Geometry: final body of the model. Coordinates: model frame, mm. Face numbers are marked on the shaded views. A direction names the side the tool comes from. Round coordinates to 2 decimals unless told otherwise and drop trailing zeros. Loops run counter-clockwise (first coordinate to the right, second up) from the corner with the lowest first, then second, coordinate; pieces in that order, holes last. Notation, with made-up numbers: (59, 22.25) -> (106, 22.25) arc R22 cw to (106, 53.25) -> close; hole circle Ø5 at (9, 76.5). An arc over 180 degrees is marked (long way). Answer in a Markdown table with one row per item.
```python
from build123d import *

# Parameters (mm, degrees)
SKETCH2_R           = 1.625
BOSS_EXTRUDE1_DEPTH = 10
SKETCH3_R           = 2.875
CUT_EXTRUDE1_DEPTH  = 1.5
SKETCH4_W           = 42
SKETCH4_H           = 5
BOSS_EXTRUDE2_DEPTH = 30
SKETCH5_W           = 42
SKETCH5_H           = 5
BOSS_EXTRUDE3_DEPTH = 8
CUT_EXTRUDE2_REACH  = 44
SKETCH6_W           = 12.701613413
SKETCH6_H           = 5
CUT_EXTRUDE3_REACH  = 7
SKETCH8_R           = 1.625
SKETCH9_R           = 2.875
CUT_EXTRUDE4_DEPTH  = 1.5
CUT_EXTRUDE5_DEPTH  = 35


with BuildPart() as part:
    # Sketch2 → Boss-Extrude1 (new body)
    with BuildSketch(Plane(origin=(0, 0, 0), x_dir=(1, 0, 0), z_dir=(0, 1, 0))):
        Polygon((-21, 4.97717469), (-21, -4.97717469), (21, -4.97717469), (21, 4.97717469), (21, 12.724438723), (-21, 12.724438723), align=None)
        with Locations((-15.475, 0.182409544)):
            Circle(SKETCH2_R, mode=Mode.SUBTRACT)
        with Locations((15.475, 0.182409544)):
            Circle(SKETCH2_R, mode=Mode.SUBTRACT)
    extrude(amount=BOSS_EXTRUDE1_DEPTH)

    # Sketch3 → Cut-Extrude1 (cut)
    with BuildSketch(Plane(origin=(0, 10, 0), x_dir=(1, 0, 0), z_dir=(0, 1, 0))):
        with Locations((-15.475, 0.182409544)):
            Circle(SKETCH3_R)
        with Locations((15.475, 0.182409544)):
            Circle(SKETCH3_R)
    extrude(amount=-CUT_EXTRUDE1_DEPTH, mode=Mode.SUBTRACT)

    # Sketch4 → Boss-Extrude2 (add)
    with BuildSketch(Plane.XZ):
        with Locations((0, -10.224438723)):
            Rectangle(SKETCH4_W, SKETCH4_H)
    extrude(amount=BOSS_EXTRUDE2_DEPTH)

    # Sketch5 → Boss-Extrude3 (add)
    with BuildSketch(Plane(origin=(0, 0, -12.724438723), x_dir=(-1, 0, 0), z_dir=(0, 0, -1))):
        with Locations((0, -27.5)):
            Rectangle(SKETCH5_W, SKETCH5_H)
    extrude(amount=BOSS_EXTRUDE3_DEPTH)

    # Sketch6 → Cut-Extrude2 (cut, up to next)
    with BuildSketch(Plane.ZY.offset(21), mode=Mode.PRIVATE) as cut_extrude2_sk1:
        with Locations((-1.373632017, 2.5)):
            Rectangle(SKETCH6_W, SKETCH6_H)
    cut_extrude2_tool1 = extrude(cut_extrude2_sk1.sketch, amount=-CUT_EXTRUDE2_REACH, mode=Mode.PRIVATE) & part.part
    add(cut_extrude2_tool1.solids().sort_by_distance((-21, 2.5, -1.373632))[0], mode=Mode.SUBTRACT)

    # Sketch8 → Cut-Extrude3 (cut, up to next)
    with BuildSketch(Plane(origin=(0, -25, 0), x_dir=(1, 0, 0), z_dir=(0, 1, 0)), mode=Mode.PRIVATE) as cut_extrude3_sk1:
        with Locations((-15.475, 16.884966607)):
            Circle(SKETCH8_R)
    cut_extrude3_tool1 = extrude(cut_extrude3_sk1.sketch, amount=-CUT_EXTRUDE3_REACH, mode=Mode.PRIVATE) & part.part
    add(cut_extrude3_tool1.solids().sort_by_distance((-15.475, -25, -16.884967))[0], mode=Mode.SUBTRACT)
    # Sketch8 → Cut-Extrude3 (cut, up to next)
    with BuildSketch(Plane(origin=(0, -25, 0), x_dir=(1, 0, 0), z_dir=(0, 1, 0)), mode=Mode.PRIVATE) as cut_extrude3_sk2:
        with Locations((15.475, 16.884966607)):
            Circle(SKETCH8_R)
    cut_extrude3_tool2 = extrude(cut_extrude3_sk2.sketch, amount=-CUT_EXTRUDE3_REACH, mode=Mode.PRIVATE) & part.part
    add(cut_extrude3_tool2.solids().sort_by_distance((15.475, -25, -16.884967))[0], mode=Mode.SUBTRACT)

    # Sketch9 → Cut-Extrude4 (cut)
    with BuildSketch(Plane(origin=(0, -25, 0), x_dir=(1, 0, 0), z_dir=(0, 1, 0))):
        with Locations((-15.475, 16.884966607)):
            Circle(SKETCH9_R)
        with Locations((15.475, 16.884966607)):
            Circle(SKETCH9_R)
    extrude(amount=-CUT_EXTRUDE4_DEPTH, mode=Mode.SUBTRACT)

    # Sketch11 → Cut-Extrude5 (cut)
    with BuildSketch(Plane(origin=(0, 10, 0), x_dir=(1, 0, 0), z_dir=(0, 1, 0))):
        Polygon((-7.795347272, -4.97717469), (-5.927938177, 12.724438723), (5.927938177, 12.724438723), (7.795347272, -4.97717469), align=None)
    extrude(amount=-CUT_EXTRUDE5_DEPTH, mode=Mode.SUBTRACT)


solid = part.part
```
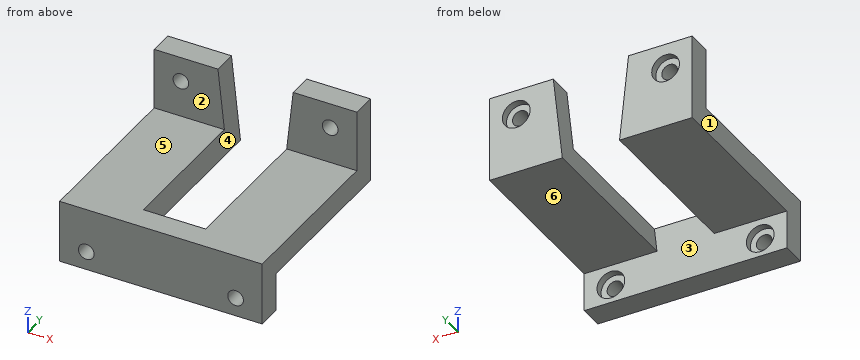
Item 1: Mould query, pull axis X, two halves, no side actions, for the marked faces 1, 2 and 3. Classes: released by +X, released by -X, zero draft, split by the parting line, or undercut.
Ans:
| item | result |
|---|---|
| face 1 | released by -X |
| face 2 | zero draft |
| face 3 | undercut |
Item 2: First-contact query: P1, Ø6.5, axis at x = -3, z = -15.5, coming from the +Y side; P2, Ø5, axis at x = -15.48, z = -0.18, coming from the +Y side; P3, Ø7.5, axis at x = -10.5, y = -8, coming from the -Z side; P4, Ø2.5, axis at x = 15.48, z = -0.18, coming from the +Y side (3 decimals). Flat tips, straight axial feed; report the tip coordinate or a pass-through.
Ans:
| item | result |
|---|---|
| P1 | y = -25 |
| P2 | y = 8.5 |
| P3 | z = -12.72 |
| P4 | through |
Item 3: Section query D-D, the plane z = -6.25. Output: boundary loops of the cut face in (x, y).
Ans:
| item | result |
|---|---|
| outline | (-21, 5) -> (-6.61, 5) -> (-6.61, 10) -> (-21, 10) -> close; (6.61, 5) -> (21, 5) -> (21, 10) -> (6.61, 10) -> close |
Item 4: Section query B-B, the plane x = 16.5. Output: boundary loops of the cut face in (y, z).
Ans:
| item | result |
|---|---|
| outline | (-30, -20.72) -> (-25, -20.72) -> (-25, -19.57) -> (-26.5, -19.57) -> (-26.5, -18.15) -> (-30, -18.15) -> close; (-30, -15.62) -> (-26.5, -15.62) -> (-26.5, -14.2) -> (-25, -14.2) -> (-25, -12.72) -> (10, -12.72) -> (10, -2.87) -> (8.5, -2.87) -> (8.5, -1.44) -> (5, -1.44) -> (5, -7.72) -> (-30, -7.72) -> close; (5, 1.08) -> (8.5, 1.08) -> (8.5, 2.5) -> (10, 2.5) -> (10, 4.98) -> (5, 4.98) -> close |
Item 5: Set-up query: the marked faces 4, 5 and 6. Return all of +Z, -Z, +X, -X, +Y, -Y with unobstructed straight access to the full face (end or side cutting, diameter ignored); none if empty.
Ans:
| item | result |
|---|---|
| face 4 | +Z, +Y |
| face 5 | +Z, +X, -X, -Y |
| face 6 | -Z, +X, -X, +Y |
Item 6: Section query C-C, the plane z = 0.5. Output: boundary loops of the cut face in (x, y), and give its area (3 significant figures).
Ans:
| item | result |
|---|---|
| outline | (-21, 5) -> (-16.95, 5) -> (-16.95, 8.5) -> (-18.27, 8.5) -> (-18.27, 10) -> (-21, 10) -> close; (-14, 5) -> (-7.32, 5) -> (-7.32, 10) -> (-12.68, 10) -> (-12.68, 8.5) -> (-14, 8.5) -> close; (7.32, 5) -> (14, 5) -> (14, 8.5) -> (12.68, 8.5) -> (12.68, 10) -> (7.32, 10) -> close; (16.95, 5) -> (21, 5) -> (21, 10) -> (18.27, 10) -> (18.27, 8.5) -> (16.95, 8.5) -> close |
| area | 99.4 mm2 |
Item 7: Section query A-A, the plane y = -22.5. Output: boundary loops of the cut face in (x, z), and give its area (3 significant figures).
Ans:
| item | result |
|---|---|
| outline | (-21, -12.72) -> (-5.93, -12.72) -> (-6.46, -7.72) -> (-21, -7.72) -> close; (5.93, -12.72) -> (21, -12.72) -> (21, -7.72) -> (6.46, -7.72) -> close |
| area | 148 mm2 |
Item 8: Ray query, L1, parallel to Y at x = 4, z = -11.25; L2, parallel to Y at x = -14, z = -1.75; L3, parallel to Z at x = -16, y = -3. Return the intervals inside material, ascending.
Ans:
| item | result |
|---|---|
| L1 | -30 to -25 |
| L2 | 5 to 8.5 |
| L3 | -12.72 to -7.72 |
